```python
from build123d import *

# Parameters (mm, degrees)
BOSS_EXTRUDE1_DEPTH = 5
SHELL1_T            = -1
BOSS_EXTRUDE2_DEPTH = 2
SKETCH3_W           = 6.8
SKETCH3_H           = 4.9
BOSS_EXTRUDE3_DEPTH = 3.5
CUT_EXTRUDE1_DEPTH  = 3.5
CUT_EXTRUDE2_DEPTH  = 1


with BuildPart() as part:
    # Sketch1 → Boss-Extrude1 (new body)
    with BuildSketch(Plane(origin=(0, 0, 0), x_dir=(1, 0, 0), z_dir=(0, 1, 0))):
        Polygon((9.025, 5.210586179), (0, 10.421172359), (-9.025, 5.210586179), (-9.025, -5.210586179), (0, -10.421172359), (9.025, -5.210586179), align=None)
    extrude(amount=BOSS_EXTRUDE1_DEPTH)

    # Shell1
    shell1_openings = [part.faces().sort_by_distance(p)[0] for p in [
        (0, 0, 0),
    ]]
    offset(amount=SHELL1_T, openings=shell1_openings, kind=Kind.INTERSECTION)

    # Sketch2 → Boss-Extrude2 (add)
    with BuildSketch(Plane.XZ.offset(-4)):
        Polygon((8.025, -4.63323591), (8.025, 4.63323591), (0, 9.26647182), (-8.025, 4.63323591), (-8.025, -4.63323591), (0, -9.26647182), align=None)
    extrude(amount=BOSS_EXTRUDE2_DEPTH)

    # Sketch3 → Boss-Extrude3 (add)
    with BuildSketch(Plane.XZ.offset(-2)):
        Rectangle(SKETCH3_W, SKETCH3_H)
    extrude(amount=BOSS_EXTRUDE3_DEPTH)

    # Sketch4 → Cut-Extrude1 (cut)
    with BuildSketch(Plane.XZ.offset(1.5)):
        Polygon((2.1, -0.65), (2.1, 0.65), (0.75, 0.65), (0.75, 2.1), (-0.75, 2.1), (-0.75, 0.65), (-2.1, 0.65), (-2.1, -0.65), (-0.75, -0.65), (-0.75, -2.1), (0.75, -2.1), (0.75, -0.65), align=None)
    extrude(amount=-CUT_EXTRUDE1_DEPTH, mode=Mode.SUBTRACT)

    # Sketch5 → Cut-Extrude2 (cut)
    with BuildSketch(Plane(origin=(0, 5, 0), x_dir=(1, 0, 0), z_dir=(0, 1, 0))):
        with BuildLine():
            Line((-5.325433461, -0.506892934), (-5.682404615, -1.575402549))
            add(Edge.make_bspline(
                [(-5.682404615, -1.575402549), (-5.738611571, -1.55146657), (-5.846580721, -1.505487433), (-6.00645553, -1.450457601), (-6.157396888, -1.414148084), (-6.299119737, -1.39335946), (-6.432402529, -1.39262203), (-6.556831326, -1.405715783), (-6.672502146, -1.438161724), (-6.741797161, -1.473664937), (-6.776154615, -1.491267934)],
                knots=[0, 0, 0, 0, 1.28771263, 2.473594846, 3.559332536, 4.55671893, 5.485823958, 6.361652317, 7.187683927, 8, 8, 8, 8], degree=3))
            add(Edge.make_bspline(
                [(-6.776154615, -1.491267934), (-6.806492545, -1.510352721), (-6.864710582, -1.546976143), (-6.938739485, -1.61588131), (-6.99599337, -1.693290765), (-7.035307029, -1.777376197), (-7.058013134, -1.861350567), (-7.065305532, -1.942177188), (-7.054051685, -2.018272363), (-7.032137808, -2.062995336), (-7.021346922, -2.085017934)],
                knots=[0, 0, 0, 0, 1.209748172, 2.321488709, 3.39707423, 4.445359682, 5.44094777, 6.3240213, 7.174710374, 8, 8, 8, 8], degree=3))
            add(Edge.make_bspline(
                [(-7.021346922, -2.085017934), (-7.007656472, -2.106037373), (-6.980319555, -2.148008721), (-6.925567054, -2.201021253), (-6.862951825, -2.247786346), (-6.815080973, -2.270504668), (-6.790577692, -2.282133319)],
                knots=[0, 0, 0, 0, 0.973157049, 1.943187581, 2.947195419, 4, 4, 4, 4], degree=3))
            add(Edge.make_bspline(
                [(-6.790577692, -2.282133319), (-6.769858792, -2.290097745), (-6.7215347, -2.308673716), (-6.63598808, -2.33053668), (-6.529832527, -2.359308535), (-6.401725396, -2.388293787), (-6.252497256, -2.421379678), (-6.081066664, -2.454151642), (-5.88849741, -2.491724711), (-5.752544005, -2.516649981), (-5.681202692, -2.529729472)],
                knots=[0, 0, 0, 0, 0.467887767, 1.091286356, 1.859988272, 2.788638217, 3.861161716, 5.084362453, 6.470024239, 8, 8, 8, 8], degree=3))
            add(Edge.make_bspline(
                [(-5.681202692, -2.529729472), (-5.614688545, -2.541707449), (-5.488466865, -2.564437657), (-5.309075132, -2.597398063), (-5.149619325, -2.624932828), (-5.010942301, -2.653591474), (-4.892650506, -2.677133355), (-4.794430155, -2.697661701), (-4.716489125, -2.714957182), (-4.671549695, -2.727498295), (-4.652356538, -2.732854472)],
                knots=[0, 0, 0, 0, 1.546287761, 2.93433875, 4.173173077, 5.24819644, 6.174012619, 6.932675225, 7.544156831, 8, 8, 8, 8], degree=3))
            add(Edge.make_bspline(
                [(-4.652356538, -2.732854472), (-4.576623584, -2.754433542), (-4.430948197, -2.795941753), (-4.228232443, -2.875630456), (-4.047908963, -2.962859498), (-3.890344122, -3.062664527), (-3.751179655, -3.17552418), (-3.624703925, -3.301019132), (-3.512720637, -3.444029872), (-3.448277986, -3.547923786), (-3.415577692, -3.600642934)],
                knots=[0, 0, 0, 0, 1.214203853, 2.335570051, 3.355534606, 4.300291848, 5.205716251, 6.114761862, 7.043368914, 8, 8, 8, 8], degree=3))
            add(Edge.make_bspline(
                [(-3.415577692, -3.600642934), (-3.386940184, -3.653439855), (-3.330617955, -3.757277112), (-3.264417801, -3.919102949), (-3.215768933, -4.082115905), (-3.185465465, -4.246531266), (-3.173372547, -4.41177459), (-3.179504364, -4.578223869), (-3.204041341, -4.745238515), (-3.244721037, -4.911960498), (-3.30204991, -5.075343685), (-3.377031051, -5.231803254), (-3.467113417, -5.380417938), (-3.574802899, -5.519417001), (-3.695616106, -5.652007924), (-3.834104159, -5.775095202), (-3.988505341, -5.889617335), (-4.100107682, -5.957675309), (-4.15716423, -5.992469857)],
                knots=[0, 0, 0, 0, 1.025678726, 2.017232489, 2.981083202, 3.927665712, 4.867989921, 5.806443481, 6.767762737, 7.747334686, 8.73460219, 9.720539785, 10.706714995, 11.69798516, 12.720254519, 13.76740984, 14.858591258, 16, 16, 16, 16], degree=3))
            add(Edge.make_bspline(
                [(-4.15716423, -5.992469857), (-4.2029151, -6.017928425), (-4.293326345, -6.068238741), (-4.43299698, -6.132088815), (-4.573498408, -6.183443266), (-4.714079103, -6.224567518), (-4.854784589, -6.256505215), (-4.996764563, -6.275817947), (-5.139055192, -6.282263566), (-5.281711595, -6.280685803), (-5.425609337, -6.265765459), (-5.571059365, -6.239249342), (-5.718130016, -6.200666559), (-5.86656675, -6.149043701), (-6.01792839, -6.088380432), (-6.170664985, -6.014503942), (-6.325132479, -5.928971262), (-6.426330514, -5.864420115), (-6.478077692, -5.831412165)],
                knots=[0, 0, 0, 0, 1.017774509, 2.011289818, 2.982347635, 3.9240255, 4.857710421, 5.785363618, 6.705792502, 7.625165849, 8.556898814, 9.514964358, 10.497515854, 11.510029584, 12.568949849, 13.666508622, 14.80677927, 16, 16, 16, 16], degree=3))
            Line((-6.478077692, -5.831412165), (-5.93841423, -4.849441011))
            add(Edge.make_bspline(
                [(-5.93841423, -4.849441011), (-5.876066943, -4.885737418), (-5.756838552, -4.955148012), (-5.576733209, -5.038518479), (-5.405875784, -5.100678252), (-5.242445562, -5.135796737), (-5.0879048, -5.149004574), (-4.941778751, -5.138495445), (-4.803236577, -5.10468289), (-4.720183882, -5.061876928), (-4.678798845, -5.04054678)],
                knots=[0, 0, 0, 0, 1.293579815, 2.47374744, 3.555769028, 4.54819344, 5.46380976, 6.3287118, 7.167199521, 8, 8, 8, 8], degree=3))
            add(Edge.make_bspline(
                [(-4.678798845, -5.04054678), (-4.638936237, -5.015446967), (-4.561347561, -4.966592631), (-4.464150913, -4.872487164), (-4.387701145, -4.765879064), (-4.334443541, -4.648855696), (-4.303317377, -4.529157536), (-4.294197846, -4.412572162), (-4.313533945, -4.301642045), (-4.345449099, -4.235867679), (-4.361491153, -4.202806396)],
                knots=[0, 0, 0, 0, 1.138617944, 2.216208663, 3.252996335, 4.299549031, 5.311698101, 6.23549815, 7.113078549, 8, 8, 8, 8], degree=3))
            add(Edge.make_bspline(
                [(-4.361491153, -4.202806396), (-4.380010417, -4.173871492), (-4.4175359, -4.115240856), (-4.4965852, -4.041680531), (-4.589626245, -3.976678965), (-4.680359291, -3.930555918), (-4.765056268, -3.897993387), (-4.843056545, -3.872966048), (-4.933757848, -3.846171338), (-5.038856401, -3.822065238), (-5.155920712, -3.794858002), (-5.286890039, -3.77045363), (-5.430568678, -3.743553698), (-5.531326246, -3.727039534), (-5.583846922, -3.718431396)],
                knots=[0, 0, 0, 0, 0.909424095, 1.84276103, 2.843738267, 3.919499091, 4.536166438, 5.253068241, 6.095165878, 7.047724124, 8.116724405, 9.287726519, 10.586206066, 12, 12, 12, 12], degree=3))
            add(Edge.make_bspline(
                [(-5.583846922, -3.718431396), (-5.683655771, -3.701485292), (-5.875498665, -3.668913133), (-6.150918918, -3.617525985), (-6.401889951, -3.56506577), (-6.628381182, -3.511091226), (-6.830571857, -3.456261035), (-7.008205883, -3.400069991), (-7.161834982, -3.344104119), (-7.293538663, -3.286043885), (-7.407482868, -3.222236129), (-7.512689732, -3.158161164), (-7.608810661, -3.087752964), (-7.698405428, -3.014463112), (-7.780415921, -2.936493879), (-7.853571897, -2.853349852), (-7.919489932, -2.766364229), (-7.956953592, -2.704748877), (-7.975673845, -2.673960242)],
                knots=[0, 0, 0, 0, 1.801703634, 3.463060095, 4.985942132, 6.364289375, 7.606258193, 8.713464438, 9.679023598, 10.515207159, 11.27148115, 12.001589174, 12.706147237, 13.389942357, 14.060675862, 14.717353214, 15.359072975, 16, 16, 16, 16], degree=3))
            add(Edge.make_bspline(
                [(-7.975673845, -2.673960242), (-7.999795613, -2.629122769), (-8.047616039, -2.540234299), (-8.103161683, -2.400567973), (-8.141164791, -2.257609045), (-8.166399838, -2.112801598), (-8.172416775, -1.965223955), (-8.166195079, -1.81528572), (-8.140455592, -1.663084625), (-8.103487814, -1.509287165), (-8.048666477, -1.358978393), (-7.983473223, -1.214192623), (-7.903174289, -1.078774796), (-7.810666895, -0.951928095), (-7.703446581, -0.834805086), (-7.584683375, -0.725513924), (-7.452816447, -0.6246676), (-7.357251696, -0.566533109), (-7.308606538, -0.536941011)],
                knots=[0, 0, 0, 0, 0.980347626, 1.943499407, 2.887156219, 3.826129841, 4.768902428, 5.727093312, 6.711776165, 7.737615518, 8.770284615, 9.789131514, 10.792512546, 11.797495335, 12.808358981, 13.846235693, 14.903673103, 16, 16, 16, 16], degree=3))
            add(Edge.make_bspline(
                [(-7.308606538, -0.536941011), (-7.243289176, -0.501983178), (-7.113314521, -0.43242078), (-6.904353926, -0.35846878), (-6.687820942, -0.308992515), (-6.500600952, -0.28813955), (-6.344609626, -0.287208489), (-6.219649665, -0.29249956), (-6.087866756, -0.309558499), (-5.948942979, -0.331728905), (-5.802667888, -0.363649134), (-5.649701479, -0.403532254), (-5.488917483, -0.449902409), (-5.38095366, -0.487538594), (-5.325433461, -0.506892934)],
                knots=[0, 0, 0, 0, 1.296925376, 2.580744562, 3.870196999, 5.183781057, 5.871953614, 6.603064647, 7.373865503, 8.19924855, 9.068280055, 9.996460477, 10.96968344, 12, 12, 12, 12], degree=3))
        make_face()
        Polygon((-4.727074029, 0.779164758), (-3.724670183, 1.357289758), (-2.592458644, -0.601844857), (-0.855679798, 0.401760912), (-1.987891337, 2.360895528), (-0.98909326, 2.937818604), (2.01090674, -2.255691011), (1.012108663, -2.832614088), (-0.302795183, -0.554969857), (-2.039574029, -1.558575626), (-0.724670183, -3.836219857), (-1.727074029, -4.414344857), align=None)
        Polygon((0.219435962, 3.634933989), (2.797560962, 5.122914758), (3.355253269, 4.158972451), (1.755493654, 3.235895528), (2.298762885, 2.293587835), (3.8985225, 3.216664758), (4.447801346, 2.267145528), (2.848041731, 1.344068604), (4.197801346, -0.99367178), (3.219435962, -1.558575626), align=None)
        Polygon((3.158297192, 5.330847451), (6.0284895, 6.988299374), (6.592191423, 6.013539758), (5.646277961, 5.467866681), (8.082576038, 1.249116681), (7.078970269, 0.669789758), (4.642672192, 4.888539758), (3.721999115, 4.356087835), align=None)
    extrude(amount=-CUT_EXTRUDE2_DEPTH, mode=Mode.SUBTRACT)


solid = part.part
```
For this review, take the finished solid that the model builds, in its own axes (mm). A direction names the side the tool comes from. Coordinates: 2 decimals unless noted, no trailing zeros. Loops run counter-clockwise (first coordinate to the right, second up) from the corner with the lowest first, then second, coordinate; pieces in that order, holes last.
1. For faces 4 (the flat face through (1, 0, 0.65)), 5 (the flat face through (3.44, 4.51, -4.84)), 6 (the flat face through (-4.45, 2.46, -7.85)), list the 3-axis set-ups (+Z, -Z, +X, -X, +Y, -Y) from which the entire face can be reached by the end or side of a thin tool; tool diameter is ignored.
2. Mouldability with a two-part tool opening along X and no side actions: class faces 1 (the flat face through (0, 5, 2)), 2 (the flat face through (3.72, 4.51, 1.27)), 3 (the flat face through (-9.025, 2, 0)) as +X half, -X half, draft (parallel to the pull), parting line (faces both ways), or undercut.
3. Insertion check: P1, Ø1.5, axis at y = -1, z = -1.5, coming from the +X side; P2, Ø9, axis at x = -1.5, z = -4.5, coming from the -Y side; P3, Ø6, axis at x = -2.5, z = 7.5, coming from the -Y side; P4, Ø2, axis at x = 0.5, y = 1.5, coming from the -Z side. Each pin has a flat end and moves straight along its axis. Give the tip position at first contact, or say it passes through.
4. Add section B-B, the plane y = -0.25. Give the boundary of the cut face in (x, z).
5. For line 1 (X direction, y = 1, z = 1.25) (3 decimals); line 2 (Z direction, x = 2.25, y = 1.25); line 3 (Z direction, x = 1.75, y = 1.25), list the stretches that pass through material, from the lowest coordinate up.
6. Add section C-C, the plane z = 7.25. Give the boundary of the cut face in (x, y).
7. Add section A-A, the plane y = 1.5. Give the boundary of the cut face in (x, z) (3 decimals), then the cut area to 3 significant figures.
8. Add section D-D, the plane y = 3.5. Give the boundary of the cut face in (x, z) (3 decimals).
Result:
1. face 4: -Y
1. face 5: +Y
1. face 6: -Z, -X, +Y, -Y
2. face 1: draft
2. face 2: undercut
2. face 3: -X half
3. P1: stops at x = 3.4
3. P2: stops at y = -1.5
3. P3: stops at y = 0
3. P4: stops at z = -10.42
4. outline: (-3.4, -2.45) - (3.4, -2.45) - (3.4, 2.45) - (-3.4, 2.45) - close; hole (-2.1, -0.65) - (-0.75, -0.65) - (-0.75, -2.1) - (0.75, -2.1) - (0.75, -0.65) - (2.1, -0.65) - (2.1, 0.65) - (0.75, 0.65) - (0.75, 2.1) - (-0.75, 2.1) - (-0.75, 0.65) - (-2.1, 0.65) - close
5. line 1: x = -9.025 to -8.025, -3.4 to -0.75, 0.75 to 3.4, 8.025 to 9.025
5. line 2: z = -9.12 to -7.97, -2.45 to 2.45, 7.97 to 9.12
5. line 3: z = -9.41 to -8.26, -2.45 to -0.65, 0.65 to 2.45, 8.26 to 9.41
6. outline: (-5.49, 0) - (-3.49, 0) - (-3.49, 2) - (3.49, 2) - (3.49, 0) - (5.49, 0) - (5.49, 5) - (-5.49, 5) - close
7. outline: (-9.025, -5.211) - (0, -10.421) - (9.025, -5.211) - (9.025, 5.211) - (0, 10.421) - (-9.025, 5.211) - close; (-3.4, -2.45) - (3.4, -2.45) - (3.4, 2.45) - (-3.4, 2.45) - close; hole (-8.025, -4.633) - (0, -9.266) - (8.025, -4.633) - (8.025, 4.633) - (0, 9.266) - (-8.025, 4.633) - close; hole (-2.1, -0.65) - (-0.75, -0.65) - (-0.75, -2.1) - (0.75, -2.1) - (0.75, -0.65) - (2.1, -0.65) - (2.1, 0.65) - (0.75, 0.65) - (0.75, 2.1) - (-0.75, 2.1) - (-0.75, 0.65) - (-2.1, 0.65) - close
7. area: 82.6 mm2
8. outline: (-9.025, -5.211) - (0, -10.421) - (9.025, -5.211) - (9.025, 5.211) - (0, 10.421) - (-9.025, 5.211) - close
